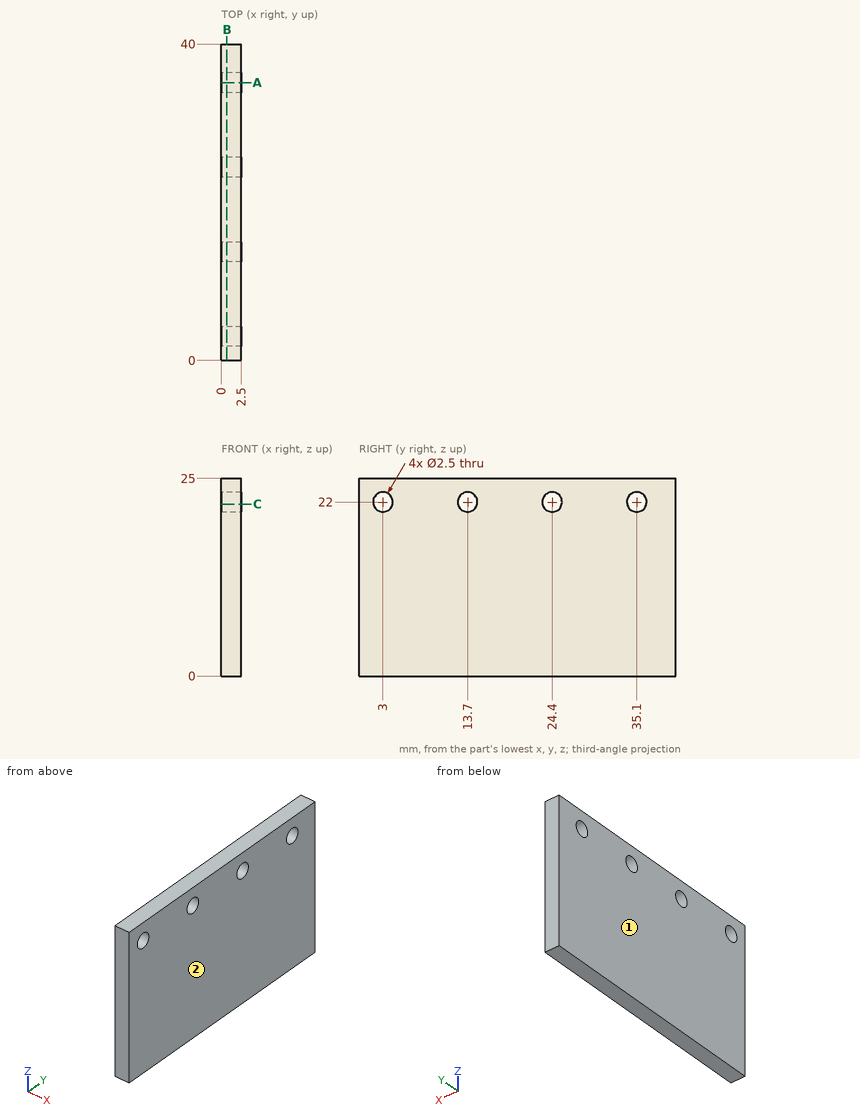
Part print with two shaded views. Sizes in mm from the minimum x, y, z corner. Give positions to 0.01 mm unless a question says otherwise; leave off trailing zeros. Order: outer loops, then holes, each group sorted by start corner. A loop starts at its lowest first (then second) coordinate and runs counter-clockwise, first axis right, second up.
1) Saw through at B-B, the plane x = 0.7. Write the cut outline in (y, z).
2) Saw through at A-A, the plane y = 35.1. Write the cut outline in (x, z).
3) Saw through at C-C, the plane z = 21.75. Write the cut outline in (x, y), then the cut area to 3 significant figures.
4) Mould opens along X. For the marked faces 1 and 2 say: +X half, -X half, draft (parallel to the pull), parting line (faces both ways), or undercut.
5) Wall check: probe 1 along Y at (x, z) = (1.75, 22); probe 2 along Z at (x, y) = (1.35, 3.5). Give the ranges that are in metal, low to high.
Computed:
1. outline: (0, 0) - (40, 0) - (40, 25) - (0, 25) - close; hole circle Ø2.5 at (3, 22); hole circle Ø2.5 at (13.7, 22); hole circle Ø2.5 at (24.4, 22); hole circle Ø2.5 at (35.1, 22)
2. outline: (0, 0) - (2.5, 0) - (2.5, 20.75) - (0, 20.75) - close; (0, 23.25) - (2.5, 23.25) - (2.5, 25) - (0, 25) - close
3. outline: (0, 0) - (2.5, 0) - (2.5, 1.78) - (0, 1.78) - close; (0, 4.22) - (2.5, 4.22) - (2.5, 12.48) - (0, 12.48) - close; (0, 14.92) - (2.5, 14.92) - (2.5, 23.18) - (0, 23.18) - close; (0, 25.62) - (2.5, 25.62) - (2.5, 33.88) - (0, 33.88) - close; (0, 36.32) - (2.5, 36.32) - (2.5, 40) - (0, 40) - close
3. area: 75.5 mm2
4. face 1: -X half
4. face 2: +X half
5. probe 1: y = 0 to 1.75, 4.25 to 12.45, 14.95 to 23.15, 25.65 to 33.85, 36.35 to 40
5. probe 2: z = 0 to 20.85, 23.15 to 25
